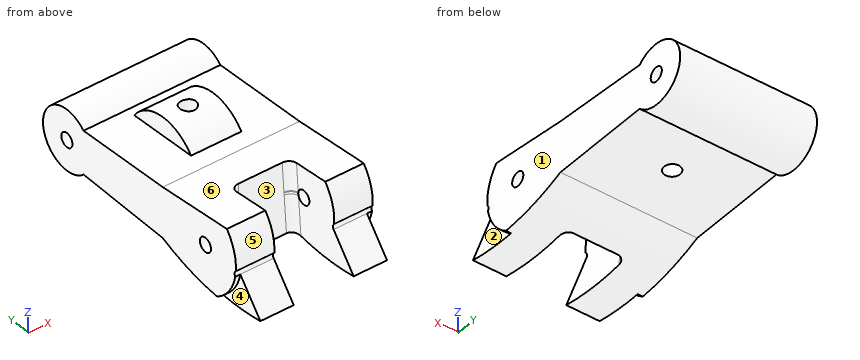
from build123d import *

# Parameters (mm, degrees)
F0_R      = 4.445
F1_DEPTH  = 43.5102
F4_DEPTH  = 16.002
F5_R      = 5.08
F6_DEPTH  = 76.2
F8_DEPTH  = 3.2512
F10_DEPTH = 48.8043176288
F11_R     = 5.08


# Not quite as in the source:
# - a pattern or mirror of a feature is missing from the dataset's text; its kind, count and spacing are read off the source's solid


with BuildPart() as f1:
    # F0 (on Right) → F1 (new body, symmetric)
    with BuildSketch(Plane.YZ):
        with BuildLine():
            Line((-20.0435682294, -15.8600244388), (43.1716607283, -13.6525))
            ThreePointArc((43.1716607283, -13.6525), (75.5074329584, 0), (43.1716607283, 13.6525))
            Line((43.1716607283, 13.6525), (-20.0435682294, 15.8600244388))
            ThreePointArc((-20.0435682294, 15.8600244388), (-15.7347770092, 0), (-20.0435682294, -15.8600244388))
        make_face()
        with Locations((56.4574329584, 0)):
            Circle(F0_R, mode=Mode.SUBTRACT)
        with BuildLine():
            ThreePointArc((-93.8586293632, -25.5824005626), (-56.2599595636, -25.9685392928), (-20.0435682294, -15.8600244388))
            ThreePointArc((-20.0435682294, -15.8600244388), (-15.7347770092, 0), (-20.0435682294, 15.8600244388))
            Line((-20.0435682294, 15.8600244388), (-71.2014077133, 20.0125123513))
            ThreePointArc((-71.2014077133, 20.0125123513), (-76.9181304267, 9.5922039668), (-78.3441527071, -2.2073810202))
            ThreePointArc((-78.3441527071, -2.2073810202), (-77.3808721828, -3.9314055649), (-77.8723212002, -5.8441647924))
            Line((-77.8723212002, -5.8441647924), (-93.8586293632, -25.5824005626))
        make_face()
        with Locations((-54.0887770092, 0)):
            Circle(F0_R, mode=Mode.SUBTRACT)
    extrude(amount=F1_DEPTH, both=True)

    # F3 (on Right) → F4 (join, symmetric)
    with BuildSketch(Plane.YZ):
        with BuildLine():
            ThreePointArc((37.2042329584, 13.8608871696), (14.9518760887, 26.202001098), (-8.1071477478, 15.4431954506))
            Line((-8.1071477478, 15.4431954506), (37.2042329584, 13.8608871696))
        make_face()
    extrude(amount=F4_DEPTH, both=True)

    # F5 (on Top) → F6 (cut, symmetric)
    with BuildSketch(Plane.XY):
        with Locations((0, 14.5474329584)):
            Circle(F5_R)
    extrude(amount=F6_DEPTH, both=True, mode=Mode.SUBTRACT)

    # F7 (on face) → F8 (cut)
    with BuildSketch(Plane.YZ.offset(43.5102)):
        with BuildLine():
            ThreePointArc((-63.4642960228, -26.7193360516), (-72.8742694492, -17.8043026874), (-77.8723212002, -5.8441647924))
            Line((-77.8723212002, -5.8441647924), (-93.8586293632, -25.5824005626))
            ThreePointArc((-93.8586293632, -25.5824005626), (-78.69393168, -27.0188799259), (-63.4642960228, -26.7193360516))
        make_face()
    f8 = extrude(amount=-F8_DEPTH, mode=Mode.SUBTRACT)

    # F8_copies: F8 across plane
    add(f8.mirror(Plane(origin=(0, 0, 0), x_dir=(0, 0, -1), z_dir=(-1, 0, 0))), mode=Mode.SUBTRACT)

    # F9 (on face) → F10 (cut, through all)
    with BuildSketch(Plane(origin=(0, 1.1477392706, 14.1399234898), x_dir=(1, 0, 0), z_dir=(0, 0.0809040348, 0.9967218956))):
        Polygon((19.05, -91.4812315527), (19.05, -44.4912315527), (0, -44.4912315527), (-19.05, -44.4912315527), (-19.05, -91.4812315527), align=None)
    extrude(amount=-F10_DEPTH, mode=Mode.SUBTRACT)

    # F11
    f11_edges = [f1.edges().sort_by_distance(p)[0] for p in [
        (19.05, -44.905298, -3.298502),
        (-19.05, -44.905298, -3.298502),
    ]]
    fillet(f11_edges, radius=F11_R)


solid = f1.part
Can you work these out from the model? Positions are in its coordinate system, mm. Face numbers are marked on the shaded views. A direction names the side the tool comes from. Give positions to 0.01 mm unless a question says otherwise; leave off trailing zeros. Write each loop counter-clockwise with the first axis right and the second up, starting at its lowest first coordinate (ties: lowest second). Pieces come first, ordered by that corner, then holes. Notation, with made-up numbers: (42, 19.5) -> (57, 19.5) arc R24 ccw to (57, 55.5) -> close; hole circle Ø4 at (-29.5, 23). An arc over 180 degrees is marked (long way). Answer as a JSON object with one key per item and string values. Group by question number.
Item 1: Suppose I cut it at A-A (x = 0). State how many separate pieces and enclosed holes the cut face has, plus the area to 3 significant figures.
Item 2: Suppose I cut it at C-C (z = 23.5). Please give me the cut outline in (x, y), plus the area to 3 significant figures.
Item 3: We'd pull the mould along Y, two halves only. Please class the marked faces 4, 5 and 6: +Y half, -Y half, draft (parallel to the pull), parting line (faces both ways), or undercut.
Item 4: Please list where these lines run through material, in increasing order: line 1 (Y direction, x = -36, z = 4); line 2 (X direction, y = -86, z = -22.5); line 3 (X direction, y = -52.5, z = 13.5). Write a range as [from, to].
Item 5: I'm going to push flat-ended pins straight in: P1, Ø4, axis at x = -3.5, y = 43, coming from the -Z side; P2, Ø12, axis at x = -27.5, y = -42, coming from the +Z side; P3, Ø1, axis at x = -13, y = -11, coming from the +Z side; P4, Ø8, axis at y = -54.09, z = 0, coming from the -X side. Where does each tip first touch, or does it pass through?
Item 6: For the marked faces 1, 2 and 3, which set-ups out of +Z, -Z, +X, -X, +Y, -Y let a thin tool reach every point of the face, with its end or its side?
Findings:
{
 "1": {"separate pieces": "2", "enclosed holes": "1", "area": "3,710 mm²"},
 "2": {"outline": "(-16, 1.94) -> (16, 1.94) -> (16, 26.01) -> (-16, 26.01) -> close; hole circle Ø10.16 at (0, 14.55)", "area": "690 mm²"},
 "3": {"face 4": "draft", "face 5": "-Y half", "face 6": "undercut"},
 "4": {"line 1": "y = [-78.17, -56.03], [-52.15, 54.52], [58.4, 75.08]", "line 2": "x = [-40.26, -19.05], [19.05, 40.26]", "line 3": "x = [-43.51, -19.05], [19.05, 43.51]"},
 "5": {"P1": "stops at z = -15.22", "P2": "stops at z = 18.13", "P3": "stops at z = 15.56", "P4": "passes through"},
 "6": {"face 1": "+Z, -Z, +X, +Y, -Y", "face 2": "-Z, +X, -Y", "face 3": "+Z, -Y"}
}
